Here's how the part is built. I have some questions about the finished solid (model axes, mm). A direction names the side the tool comes from. Round coordinates to 2 decimals unless told otherwise and drop trailing zeros. Loops run counter-clockwise (first coordinate to the right, second up) from the corner with the lowest first, then second, coordinate; pieces in that order, holes last. Notation, with made-up numbers: M -36.75,-23.5 L 13.25,-23.5 A8 ccw 13.25,-15.5 Z; hole C 17.25,-21.75 d3. An arc over 180 degrees is marked long. Use a Markdown table: item, result.
```python
from build123d import *

# Parameters (mm, degrees)
SKETCH3_R           = 14
SKETCH3_R_2         = 10.5
BOSS_EXTRUDE2_DEPTH = 56
SKETCH3_4_R         = 14
SKETCH3_4_R_2       = 10.5
CUT_EXTRUDE1_DEPTH  = 16
CHAMFER1_SIZE       = 1
CUT_EXTRUDE2_DEPTH  = 16


with BuildPart() as part:
    # Sketch3 → Boss-Extrude2 (new body)
    # profile 1 of 2: a face of its own
    with BuildSketch(Plane(origin=(0, 0, 0), x_dir=(1, 0, 0), z_dir=(0, 1, 0))):
        with Locations(Location((0, 0, 0), (0, 0, 270))):
            Circle(SKETCH3_R)
        Circle(SKETCH3_R_2, mode=Mode.SUBTRACT)
    # profile 2 of 2: a face of its own
    with BuildSketch(Plane(origin=(0, 0, 0), x_dir=(1, 0, 0), z_dir=(0, 1, 0))):
        Circle(SKETCH3_R_2)
    extrude(amount=BOSS_EXTRUDE2_DEPTH)

    # Sketch3_4 → Cut-Extrude1 (cut)
    with BuildSketch(Plane(origin=(0, 0, 0), x_dir=(1, 0, 0), z_dir=(0, 1, 0))):
        with Locations(Location((0, 0, 0), (0, 0, 270))):
            Circle(SKETCH3_4_R)
        with Locations(Location((0, 0, 0), (0, 0, 270))):
            Circle(SKETCH3_4_R_2, mode=Mode.SUBTRACT)
    extrude(amount=CUT_EXTRUDE1_DEPTH, mode=Mode.SUBTRACT)

    # Chamfer1
    chamfer1_edges = [part.edges().sort_by_distance(p)[0] for p in [
        (0, 56, -14),
        (0, 16, -14),
        (0, 0, -10.5),
    ]]
    chamfer(chamfer1_edges, length=CHAMFER1_SIZE)

    # Sketch5 → Cut-Extrude2 (cut)
    with BuildSketch(Plane.XY.offset(7.5)):
        with BuildLine():
            Line((-3, 5), (-3, 12))
            ThreePointArc((-3, 12), (0, 15), (3, 12))
            Line((3, 12), (3, 5))
            ThreePointArc((3, 5), (0, 2), (-3, 5))
        make_face()
    extrude(amount=CUT_EXTRUDE2_DEPTH, mode=Mode.SUBTRACT)


solid = part.part
```
Q1. Imagine slicing it at C-C, the plane y = 31. Please give me the cut outline in (x, z).
Return value:
| item | result |
|---|---|
| outline | C 0,0 d28 |
Q2. I need wall thicknesses on line 1 (Y direction, x = 1, z = 7.75); line 2 (X direction, y = 35.5, z = -3); line 3 (Z direction, x = 13, y = 32). Which ranges of each line are inside material? Lowest first, please. Write a range as from..to.
Return value:
| item | result |
|---|---|
| line 1 | y = 0..2.17, 14.83..56 |
| line 2 | x = -13.67..13.67 |
| line 3 | z = -5.2..5.2 |
Q3. For faces 5 (the flat face through (0, 56, 0)), 6 (the cylindrical face through (3.2, 8.4, 10)), 7 (the flat face through (0, 9, 7.5)), which set-ups out of +Z, -Z, +X, -X, +Y, -Y let a thin tool reach every point of the face, with its end or its side?
Return value:
| item | result |
|---|---|
| face 5 | +Z, -Z, +X, -X, +Y |
| face 6 | -Y |
| face 7 | +Z |
Q4. Imagine slicing it at B-B, the plane x = 0. Please give me the cut outline in (y, z), then the cut area to 3 significant figures.
Return value:
| item | result |
|---|---|
| outline | M 0,-9.5 L 1,-10.5 L 16,-10.5 L 16,-13 L 17,-14 L 55,-14 L 56,-13 L 56,13 L 55,14 L 17,14 L 16,13 L 16,10.5 L 15,10.5 L 15,7.5 L 2,7.5 L 2,10.5 L 1,10.5 L 0,9.5 Z |
| area | 1,410 mm^2 |
Q5. We'd pull the mould along Y, two halves only. Please class faces 1 (the cylindrical face through (0, 15, 9)), 2 (the cylindrical face through (0, 2, 9)), 3 (the flat face through (6, 16, -9)), 4 (the cylindrical face through (-13.67, 35.73, -3.03)): pulls with the +Y half, pulls with the -Y half, needs draft (parallel to the pull), parting line crosses it, or undercut.
Return value:
| item | result |
|---|---|
| face 1 | undercut |
| face 2 | undercut |
| face 3 | pulls with the -Y half |
| face 4 | needs draft |
Q6. Imagine slicing it at A-A, the plane z = 0. Please give me the cut outline in (x, y).
Return value:
| item | result |
|---|---|
| outline | M -14,17 L -13,16 L -10.5,16 L -10.5,1 L -9.5,0 L 9.5,0 L 10.5,1 L 10.5,16 L 13,16 L 14,17 L 14,55 L 13,56 L -13,56 L -14,55 Z |
Q7. Will these pins go through, and if not, where does the flat tip stop? P1, Ø5, axis at x = 0, y = 6.5, coming from the +Z side; P2, Ø4, axis at y = 20.5, z = -6.5, coming from the +X side; P3, Ø10, axis at y = 32, z = 10, coming from the -X side.
Return value:
| item | result |
|---|---|
| P1 | stops at z = 7.5 |
| P2 | stops at x = 13.26 |
| P3 | stops at x = -13.08 |
